Source: three-view drawing plus pictorial views. Frame: mm from the lowest corner of the part. Round coordinates to 2 decimals unless told otherwise and drop trailing zeros. Loops run counter-clockwise (first coordinate to the right, second up) from the corner with the lowest first, then second, coordinate; pieces in that order, holes last. Notation, with made-up numbers: (42, 17) -> (87, 17) arc R31 cw to (87, 41) -> close; hole circle Ø1 at (-28.75, -17). An arc over 180 degrees is marked (long way). Answer in a Markdown table with one row per item.
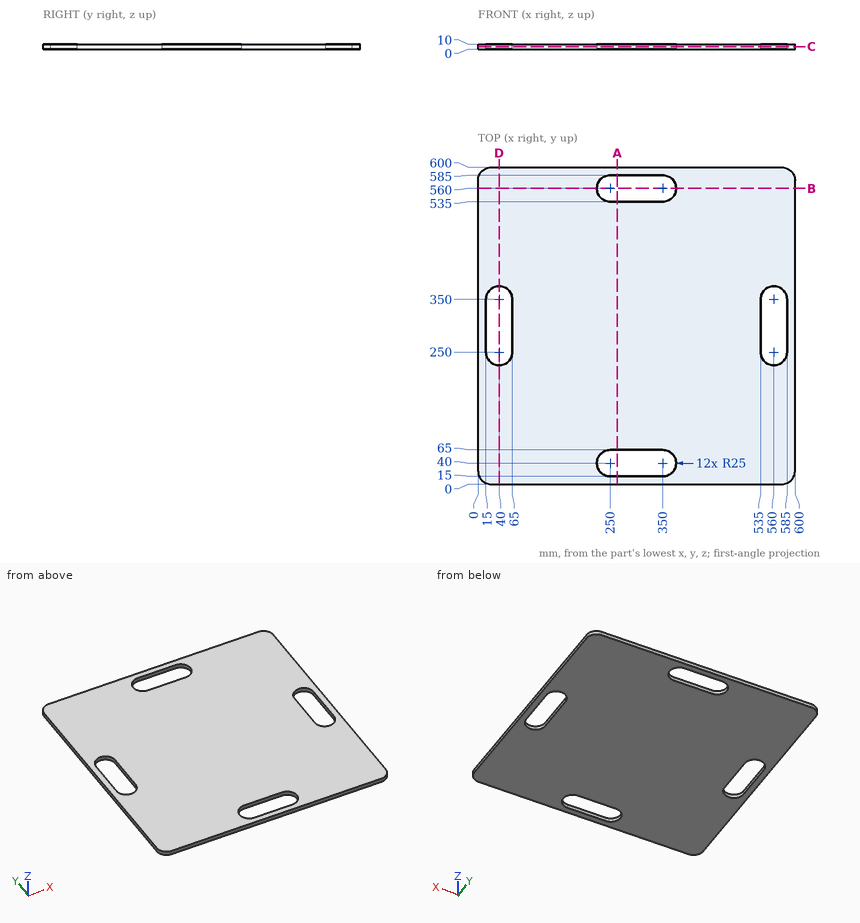
Item 1: Cut plane B-B (y = 560). Output: boundary loops of the cut face in (x, z), then the cut area to 3 significant figures.
Answer:
| item | result |
|---|---|
| outline | (0, 0) -> (225, 0) -> (225, 10) -> (0, 10) -> close; (375, 0) -> (600, 0) -> (600, 10) -> (375, 10) -> close |
| area | 4,500 mm² |
Item 2: Line query: probe 1 along Y at (x, z) = (264, 9.25); probe 2 along X at (y, z) = (59.5, 7). Output: solid intervals per line, ascending. Write a range as [from, to].
Answer:
| item | result |
|---|---|
| probe 1 | y = [0, 15], [65, 535], [585, 600] |
| probe 2 | x = [0, 234.36], [365.64, 600] |
Item 3: Cut plane C-C (z = 5). Output: boundary loops of the cut face in (x, y).
Answer:
| item | result |
|---|---|
| outline | (0, 25) arc R25 ccw to (25, 0) -> (575, 0) arc R25 ccw to (600, 25) -> (600, 575) arc R25 ccw to (575, 600) -> (25, 600) arc R25 ccw to (0, 575) -> close; hole (15, 250) arc R25 ccw to (65, 250) -> (65, 350) arc R25 ccw to (15, 350) -> close; hole (250, 15) -> (350, 15) arc R25 ccw to (350, 65) -> (250, 65) arc R25 ccw to start; hole (250, 535) -> (350, 535) arc R25 ccw to (350, 585) -> (250, 585) arc R25 ccw to start; hole (535, 250) arc R25 ccw to (585, 250) -> (585, 350) arc R25 ccw to (535, 350) -> close |
Item 4: Cut plane A-A (x = 264). Output: boundary loops of the cut face in (y, z).
Answer:
| item | result |
|---|---|
| outline | (0, 0) -> (15, 0) -> (15, 10) -> (0, 10) -> close; (65, 0) -> (535, 0) -> (535, 10) -> (65, 10) -> close; (585, 0) -> (600, 0) -> (600, 10) -> (585, 10) -> close |
